```python
from build123d import *

# Parameters (mm, degrees)
CROQUIS1_R                   = 105
SALIENTE_EXTRUIR1_DEPTH      = 3
CORTAR_EXTRUIR1_START        = -3
CORTAR_EXTRUIR1_DEPTH        = 3
REDONDEO1_R                  = 10
CROQUIS6_R                   = 1.5
CORTAR_EXTRUIR10_DEPTH       = 149.522725677
CROQUIS12_W                  = 31
CROQUIS12_H                  = 32.5
CROQUIS12_W_2                = 36
CROQUIS12_H_2                = 23
CORTAR_EXTRUIR13_DEPTH       = 149.522725677
CROQUIS16_R                  = 1.5
CORTAR_EXTRUIR16_DEPTH       = 149.522725677
CORTAR_EXTRUIR_L_MINA2_DEPTH = 10
CROQUIS18_R                  = 5
CROQUIS18_R_2                = 10
CROQUIS18_W                  = 40
CROQUIS18_H                  = 20
CROQUIS18_W_2                = 10
CROQUIS18_H_2                = 55
CORTAR_EXTRUIR17_DEPTH       = 149.522725677
REDONDEO2_R                  = 5
REDONDEO3_R                  = 10
CROQUIS19_R                  = 2
CORTAR_EXTRUIR18_DEPTH       = 149.522725677
CROQUIS20_R                  = 2
CORTAR_EXTRUIR19_DEPTH       = 149.522725677
CROQUIS21_W                  = 36
CROQUIS21_H                  = 12
CORTAR_EXTRUIR20_DEPTH       = 149.522725677


# Some blends are built 0.0001 mm under size
with BuildPart() as part:
    # Croquis1 → Saliente-Extruir1 (new body)
    with BuildSketch(Plane(origin=(0, 0, 0), x_dir=(1, 0, 0), z_dir=(0, 1, 0))):
        with Locations(Location((0, 0, 0), (0, 0, 270))):
            Circle(CROQUIS1_R)
    extrude(amount=SALIENTE_EXTRUIR1_DEPTH)

    # Croquis2 → Cortar-Extruir1 (cut)
    with BuildSketch(Plane(origin=(0, 3, 0), x_dir=(1, 0, 0), z_dir=(0, 1, 0)).offset(CORTAR_EXTRUIR1_START)):
        with BuildLine():
            ThreePointArc((35.71668902, 98.738635424), (0, 68.738635424), (-35.71668902, 98.738635424))
            ThreePointArc((-35.71668902, 98.738635424), (0, 105), (35.71668902, 98.738635424))
        make_face()
    extrude(amount=CORTAR_EXTRUIR1_DEPTH, mode=Mode.SUBTRACT)

    # Redondeo1
    redondeo1_edges = [part.edges().sort_by_distance(p)[0] for p in [
        (-35.71668902, 1.5, -98.738635424),
        (35.71668902, 1.5, -98.738635424),
    ]]
    fillet(redondeo1_edges, radius=REDONDEO1_R)

    # Croquis6 → Cortar-Extruir10 (cut, through all)
    with BuildSketch(Plane(origin=(0, 3, 0), x_dir=(1, 0, 0), z_dir=(0, 1, 0))):
        with Locations(Location((-50.7, -50, 0), (0, 0, 270))):
            Circle(CROQUIS6_R)
        with Locations(Location((-27.5, -50, 0), (0, 0, 270))):
            Circle(CROQUIS6_R)
        with Locations(Location((-50.7, -0.7, 0), (0, 0, 270))):
            Circle(CROQUIS6_R)
        with Locations(Location((-27.5, -0.7, 0), (0, 0, 270))):
            Circle(CROQUIS6_R)
        with Locations(Location((50.7, -0.7, 0), (0, 0, 270))):
            Circle(CROQUIS6_R)
        with Locations(Location((50.7, -50, 0), (0, 0, 270))):
            Circle(CROQUIS6_R)
        with Locations(Location((27.5, -50, 0), (0, 0, 270))):
            Circle(CROQUIS6_R)
        with Locations(Location((27.5, -0.7, 0), (0, 0, 270))):
            Circle(CROQUIS6_R)
        with Locations(Location((-24.6, 38, 0), (0, 0, 270))):
            Circle(CROQUIS6_R)
        with Locations(Location((-24.6, 61.2, 0), (0, 0, 270))):
            Circle(CROQUIS6_R)
        with Locations(Location((24.7, 38, 0), (0, 0, 270))):
            Circle(CROQUIS6_R)
        with Locations(Location((24.7, 61.2, 0), (0, 0, 270))):
            Circle(CROQUIS6_R)
    extrude(amount=-CORTAR_EXTRUIR10_DEPTH, mode=Mode.SUBTRACT)

    # Croquis12 → Cortar-Extruir13 (cut, through all)
    with BuildSketch(Plane(origin=(0, 3, 0), x_dir=(1, 0, 0), z_dir=(0, 1, 0))):
        with Locations((0, -52.516645147)):
            Rectangle(CROQUIS12_W, CROQUIS12_H)
        with Locations((0, -21.266645147)):
            Rectangle(CROQUIS12_W_2, CROQUIS12_H_2)
    extrude(amount=-CORTAR_EXTRUIR13_DEPTH, mode=Mode.SUBTRACT)

    # Croquis16 → Cortar-Extruir16 (cut, through all)
    with BuildSketch(Plane(origin=(0, 3, 0), x_dir=(1, 0, 0), z_dir=(0, 1, 0))):
        with Locations(Location((-19, -71.766645147, 0), (0, 0, 270))):
            Circle(CROQUIS16_R)
        with Locations(Location((20, -71.766645147, 0), (0, 0, 270))):
            Circle(CROQUIS16_R)
        with Locations(Location((-73.426669568, 19, 0), (0, 0, 270))):
            Circle(CROQUIS16_R)
        with Locations(Location((-73.426669568, -20, 0), (0, 0, 270))):
            Circle(CROQUIS16_R)
        with Locations(Location((73.426669568, 19, 0), (0, 0, 90))):
            Circle(CROQUIS16_R)
        with Locations(Location((73.426669568, -20, 0), (0, 0, 90))):
            Circle(CROQUIS16_R)
    extrude(amount=-CORTAR_EXTRUIR16_DEPTH, mode=Mode.SUBTRACT)

    # Croquis17 → Cortar-Extruir-Lámina2 (cut)
    with BuildSketch(Plane(origin=(0, 3, 0), x_dir=(1, 0, 0), z_dir=(0, 1, 0))):
        with BuildLine():
            ThreePointArc((-78.885993687, -39), (-56.815148476, -67.201479921), (-25.335426507, -84.274053917))
            Line((-25.335426507, -84.274053917), (-28.214452247, -93.850650954))
            ThreePointArc((-28.214452247, -93.850650954), (-63.271415348, -74.838011731), (-87.850311152, -43.431818182))
            Line((-87.850311152, -43.431818182), (-78.885993687, -39))
        make_face()
        with BuildLine():
            ThreePointArc((26.278435016, -83.984783462), (57.19088172, -66.882008404), (78.885993687, -39))
            Line((78.885993687, -39), (87.850311152, -43.431818182))
            ThreePointArc((87.850311152, -43.431818182), (63.689845552, -74.482236631), (29.264620814, -93.528508855))
            Line((29.264620814, -93.528508855), (26.278435016, -83.984783462))
        make_face()
    extrude(amount=-CORTAR_EXTRUIR_L_MINA2_DEPTH, mode=Mode.SUBTRACT)

    # Croquis18 → Cortar-Extruir17 (cut, through all)
    with BuildSketch(Plane(origin=(0, 3, 0), x_dir=(1, 0, 0), z_dir=(0, 1, 0))):
        with Locations(Location((-35, -73.047929471, 0), (0, 0, 270))):
            Circle(CROQUIS18_R)
        with Locations(Location((-68.583851236, -43.095885531, 0), (0, 0, 270))):
            Circle(CROQUIS18_R)
        with Locations(Location((35, -73.047929471, 0), (0, 0, 90))):
            Circle(CROQUIS18_R)
        with Locations(Location((68.583851236, -43.095885531, 0), (0, 0, 90))):
            Circle(CROQUIS18_R)
        with Locations(Location((-48, 74, 0), (0, 0, 270))):
            Circle(CROQUIS18_R_2)
        with Locations(Location((48, 74, 0), (0, 0, 270))):
            Circle(CROQUIS18_R_2)
        with Locations((0, 10.233354853)):
            Rectangle(CROQUIS18_W, CROQUIS18_H)
        with Locations((-63.583851236, -4.595885531)):
            Rectangle(CROQUIS18_W_2, CROQUIS18_H_2)
        with Locations((63.583851236, -4.595885531)):
            Rectangle(CROQUIS18_W_2, CROQUIS18_H_2)
    extrude(amount=-CORTAR_EXTRUIR17_DEPTH, mode=Mode.SUBTRACT)

    # Redondeo2
    redondeo2_edges = [part.edges().sort_by_distance(p)[0] for p in [
        (20, 1.5, -0.233354853),
        (20, 1.5, -20.233354853),
        (-20, 1.5, -0.233354853),
        (-20, 1.5, -20.233354853),
        (68.583851236, 1.5, 32.095885531),
        (58.583851236, 1.5, 32.095885531),
        (68.583851236, 1.5, -22.904114469),
        (58.583851236, 1.5, -22.904114469),
        (-58.583851236, 1.5, 32.095885531),
        (-68.583851236, 1.5, 32.095885531),
        (-58.583851236, 1.5, -22.904114469),
        (-68.583851236, 1.5, -22.904114469),
    ]]
    fillet(redondeo2_edges, radius=REDONDEO2_R - 0.0001)  # a hair under: the kernel refuses the full size

    # Redondeo3
    # the kernel refuses this fillet: 10 mm, written as the material it adds along each edge
    with BuildSketch(Plane(origin=(87.850311152, 3, 43.431818182), x_dir=(-0.49339949863850674, 0, 0.8698028137131256), z_dir=(0, -1, 0)), Plane(origin=(-28.214452247, 3, 93.850650954), x_dir=(-0.9397545440307068, 0, -0.3418499626643806), z_dir=(0, -1, 0))) as redondeo3_piece_1:
        with BuildLine():
            CenterArc((10.568181818, 9.983845423), REDONDEO3_R, 180, 93.257196161)
            Line((0.568181818, 9.983845423), (0.368181818, 9.983845423))
            ThreePointArc((0.368181818, 9.983845423), (0.084414001, 5.003286348), (-0.199676908, 0.011363636))
            Line((-0.199676908, 0.011363636), (-0.011363636, -0.199676908))
            ThreePointArc((-0.011363636, -0.199676908), (5.568181818, -0.358314859), (11.147727273, -0.199676908))
            Line((11.147727273, -0.199676908), (11.136363636, 0))
        make_face()
    extrude(amount=3)
    with BuildSketch(Plane(origin=(29.264620814, 3, 93.528508855), x_dir=(0.9358638260686325, 0, -0.35236188649764677), z_dir=(0, -1, 0)), Plane(origin=(-87.850311152, 3, 43.431818182), x_dir=(0.4933994986385089, 0, 0.8698028137131243), z_dir=(0, -1, 0))) as redondeo3_piece_2:
        with BuildLine():
            CenterArc((10.568181818, -9.983845423), REDONDEO3_R, 86.742803839, 93.257196161)
            Line((0.568181818, -9.983845423), (0.368181818, -9.983845423))
            ThreePointArc((0.368181818, -9.983845423), (0.084414001, -5.003286348), (-0.199676908, -0.011363636))
            Line((-0.199676908, -0.011363636), (-0.011363636, 0.199676908))
            ThreePointArc((-0.011363636, 0.199676908), (5.568181818, 0.358314859), (11.147727273, 0.199676908))
            Line((11.147727273, 0.199676908), (11.136363636, 0))
        make_face()
    extrude(amount=3)

    # Croquis19 → Cortar-Extruir18 (cut, through all)
    with BuildSketch(Plane(origin=(0, 3, 0), x_dir=(1, 0, 0), z_dir=(0, 1, 0))):
        with Locations(Location((-100.967732044, -2.552858359, 0), (0, 0, 270))):
            Circle(CROQUIS19_R)
        with Locations(Location((-52.694706213, 86.164191734, 0), (0, 0, 270))):
            Circle(CROQUIS19_R)
        with Locations(Location((48.273025831, 88.717050092, 0), (0, 0, 270))):
            Circle(CROQUIS19_R)
        with Locations(Location((100.967732044, 2.552858359, 0), (0, 0, 270))):
            Circle(CROQUIS19_R)
        with Locations(Location((52.694706213, -86.164191734, 0), (0, 0, 270))):
            Circle(CROQUIS19_R)
        with Locations(Location((-48.273025831, -88.717050092, 0), (0, 0, 270))):
            Circle(CROQUIS19_R)
    extrude(amount=-CORTAR_EXTRUIR18_DEPTH, mode=Mode.SUBTRACT)

    # Croquis20 → Cortar-Extruir19 (cut, through all)
    with BuildSketch(Plane(origin=(0, 3, 0), x_dir=(1, 0, 0), z_dir=(0, 1, 0))):
        with Locations(Location((-47.5, -56, 0), (0, 0, 270))):
            Circle(CROQUIS20_R)
        with Locations(Location((46.5, -56, 0), (0, 0, 90))):
            Circle(CROQUIS20_R)
        with Locations(Location((45, 58.5, 0), (0, 0, 270))):
            Circle(CROQUIS20_R)
        with Locations(Location((-45, 58.5, 0), (0, 0, 270))):
            Circle(CROQUIS20_R)
    extrude(amount=-CORTAR_EXTRUIR19_DEPTH, mode=Mode.SUBTRACT)

    # Croquis21 → Cortar-Extruir20 (cut, through all)
    with BuildSketch(Plane(origin=(0, 3, 0), x_dir=(1, 0, 0), z_dir=(0, 1, 0))):
        with Locations((0, -3.766645147)):
            Rectangle(CROQUIS21_W, CROQUIS21_H)
    extrude(amount=-CORTAR_EXTRUIR20_DEPTH, mode=Mode.SUBTRACT)


solid = part.part
```
Geometry: final body of the model. Coordinates: model frame, mm. Round coordinates to 2 decimals unless told otherwise and drop trailing zeros. Order: outer loops, then holes, each group sorted by start corner. A loop starts at its lowest first (then second) coordinate and runs counter-clockwise, first axis right, second up. Notation, with made-up numbers: (46, 34.25) -> (81, 34.25) arc R10 cw to (81, 45.25) -> close; hole circle Ø1 at (-15.5, 13). An arc over 180 degrees is marked (long way). Use one line per item in the form item = value. Start each with the question number.
1. Cut plane B-B (z = 61.5). Return the cut outline in (x, y).
2. Line query: probe 1 along Z at (x, y) = (-61, 1.6); probe 2 along X at (y, z) = (0.5, 84.5); probe 3 along X at (y, z) = (2.55, -17). Output: solid intervals per line, ascending.
3. Cut plane C-C (y = 1.75). Count the separate pieces of the cut face and the enclosed holes in it, then the cut area to 3 significant figures.
4. Pin query (flat end, axial travel): pin 1 Ø4.5 at (x, z) = (-47.5, 56) entering from -Y; pin 2 Ø1 at (x, y) = (-68, 2) entering from +Z; pin 3 Ø1 at (y, z) = (2, 13) entering from +X; pin 4 Ø1.5 at (y, z) = (1, -11.5) entering from -X. Return the tip coordinate at first contact, or that it passes through.
5. Draft query along Z for faces 1 (the face through (-18.496, 1.479, -18.808)), 2 (the face through (-20, 3, 9)), 3 (the face through (71.63, 1.52, 47.06)). Return one class per face: pulls with the +Z half, pulls with the -Z half, needs draft (parallel to the pull), parting line crosses it, or undercut.
6. Cut plane D-D (z = -27.5). Return the cut outline in (x, y).
7. Cut plane A-A (x = -12). Return the cut outline in (y, z), then the cut area to 3 significant figures.
Solution:
q1.outline = (-85.1, 0) -> (-76.3, 0) -> (-76.3, 3) -> (-85.1, 3) -> close; (-62.94, 0) -> (-15.5, 0) -> (-15.5, 3) -> (-62.94, 3) -> close; (15.5, 0) -> (62.94, 0) -> (62.94, 3) -> (15.5, 3) -> close; (76.3, 0) -> (85.1, 0) -> (85.1, 3) -> (76.3, 3) -> close
q2.probe_1 = -85.46 to -22.18, 31.38 to 63.43, 76.7 to 85.46
q2.probe_2 = -62.33 to -49.64, -25.42 to 26.49, 49.64 to 51.59, 53.8 to 62.33
q2.probe_3 = -103.61 to -68.58, -58.58 to -19.68, 19.68 to 58.58, 68.58 to 103.61
q3.separate_pieces = 1
q3.enclosed_holes = 40
q3.area = 26,000 mm^2
q4.pin_1 = 0
q4.pin_2 = 80.43
q4.pin_3 = 104.25
q4.pin_4 = -104.45
q5.face_1 = undercut
q5.face_2 = needs draft
q5.face_3 = undercut
q6.outline = (-101.33, 0) -> (101.33, 0) -> (101.33, 3) -> (-101.33, 3) -> close
q7.outline = (0, -70.78) -> (3, -70.78) -> (3, -20.23) -> (0, -20.23) -> close; (0, 32.77) -> (3, 32.77) -> (3, 36.27) -> (0, 36.27) -> close; (0, 68.77) -> (3, 68.77) -> (3, 104.31) -> (0, 104.31) -> close
q7.area = 269 mm^2
